```python
from build123d import *

# Parameters (mm, degrees)
F1_DEPTH      = 5
F3_DEPTH      = 10
F5_DEPTH      = 25
F7_R          = 6.7597979746
F6_R          = 2
F8_DEPTH      = 69.4
F9_R          = 5
F10_R         = 5
F11_T1_DEPTH  = 44.2
F11_T3_DEPTH  = 44.2
F12_T1_DEPTH  = 54.4
F12_T3_DEPTH  = 30
F12_T5_DEPTH  = 38
F12_S9_W      = 5
F12_S9_H      = 5
F12_T10_DEPTH = 5
F12_S15_W     = 5
F12_S15_H     = 5
F12_T16_DEPTH = 5
F12_S21_W     = 5
F12_S21_H     = 5
F12_T22_DEPTH = 5
F12_S27_W     = 5
F12_S27_H     = 5
F12_T28_DEPTH = 5
F12_T32_ANGLE = 90
F12_T34_ANGLE = 90


# Not quite as in the source:
# - a fillet or chamfer that OpenCascade refuses, or shapes differently, is made with other operations: its cross-section is extruded or revolved along the edge and cut away or added


with BuildPart() as f1:
    # F0 (on Front) → F1 (new body)
    with BuildSketch(Plane.XZ):
        with BuildLine():
            Line((32.2, -24), (32.2, 24))
            Line((32.2, 24), (8, 24))
            Line((8, 24), (8, 10.8))
            Line((8, 10.8), (8.4, 10.8))
            Line((8.4, 10.8), (8.4, 14.8))
            ThreePointArc((8.4, 14.8), (14.9, 21.3), (21.4, 14.8))
            Line((21.4, 14.8), (21.4, 10.8))
            Line((21.4, 10.8), (24.4, 10.8))
            Line((24.4, 10.8), (24.4, -10.8))
            Line((24.4, -10.8), (21.4, -10.8))
            Line((21.4, -10.8), (21.4, -14.8))
            ThreePointArc((21.4, -14.8), (14.9, -21.3), (8.4, -14.8))
            Line((8.4, -14.8), (8.4, -10.8))
            Line((8.4, -10.8), (-8.4, -10.8))
            Line((-8.4, -10.8), (-8.4, -14.8))
            ThreePointArc((-8.4, -14.8), (-14.9, -21.3), (-21.4, -14.8))
            Line((-21.4, -14.8), (-21.4, -10.8))
            Line((-21.4, -10.8), (-24.4, -10.8))
            Line((-24.4, -10.8), (-24.4, 10.8))
            Line((-24.4, 10.8), (-21.4, 10.8))
            Line((-21.4, 10.8), (-21.4, 14.8))
            ThreePointArc((-21.4, 14.8), (-14.9, 21.3), (-8.4, 14.8))
            Line((-8.4, 14.8), (-8.4, 10.8))
            Line((-8.4, 10.8), (-8, 10.8))
            Line((-8, 10.8), (-8, 24))
            Line((-8, 24), (-32.2, 24))
            Line((-32.2, 24), (-32.2, -24))
            Line((-32.2, -24), (32.2, -24))
        make_face()
    extrude(amount=F1_DEPTH)

    # F2 (on face) → F3 (join)
    with BuildSketch(Plane(origin=(0, 0, 0), x_dir=(-1, 0, 0), z_dir=(0, 1, 0))):
        with BuildLine():
            Line((24.4, 10.8), (24.4, -10.8))
            Line((24.4, -10.8), (21.4, -10.8))
            Line((21.4, -10.8), (21.4, -14.8))
            ThreePointArc((21.4, -14.8), (14.9, -21.3), (8.4, -14.8))
            Line((8.4, -14.8), (8.4, -10.8))
            Line((8.4, -10.8), (-8.4, -10.8))
            Line((-8.4, -10.8), (-8.4, -14.8))
            ThreePointArc((-8.4, -14.8), (-14.9, -21.3), (-21.4, -14.8))
            Line((-21.4, -14.8), (-21.4, -10.8))
            Line((-21.4, -10.8), (-24.4, -10.8))
            Line((-24.4, -10.8), (-24.4, 10.8))
            Line((-24.4, 10.8), (-21.4, 10.8))
            Line((-21.4, 10.8), (-21.4, 14.8))
            ThreePointArc((-21.4, 14.8), (-14.9, 21.3), (-8.4, 14.8))
            Line((-8.4, 14.8), (-8.4, 10.8))
            Line((-8.4, 10.8), (-8, 10.8))
            Line((-8, 10.8), (-8, 24))
            Line((-8, 24), (-32.2, 24))
            Line((-32.2, 24), (-32.2, -24))
            Line((-32.2, -24), (32.2, -24))
            Line((32.2, -24), (32.2, 24))
            Line((32.2, 24), (8, 24))
            Line((8, 24), (8, 10.8))
            Line((8, 10.8), (8.4, 10.8))
            Line((8.4, 10.8), (8.4, 14.8))
            ThreePointArc((8.4, 14.8), (14.9, 21.3), (21.4, 14.8))
            Line((21.4, 14.8), (21.4, 10.8))
            Line((21.4, 10.8), (24.4, 10.8))
        make_face()
        with BuildLine():
            Line((21.4, -14.8), (21.4, -10.8))
            Line((21.4, -10.8), (8.4, -10.8))
            Line((8.4, -10.8), (8.4, -14.8))
            ThreePointArc((8.4, -14.8), (14.9, -21.3), (21.4, -14.8))
        make_face()
        with BuildLine():
            Line((-8.4, -14.8), (-8.4, -10.8))
            Line((-8.4, -10.8), (-21.4, -10.8))
            Line((-21.4, -10.8), (-21.4, -14.8))
            ThreePointArc((-21.4, -14.8), (-14.9, -21.3), (-8.4, -14.8))
        make_face()
        with BuildLine():
            Line((8.4, 10.8), (21.4, 10.8))
            Line((21.4, 10.8), (21.4, 14.8))
            ThreePointArc((21.4, 14.8), (14.9, 21.3), (8.4, 14.8))
            Line((8.4, 14.8), (8.4, 10.8))
        make_face()
        with BuildLine():
            Line((-21.4, 10.8), (-8.4, 10.8))
            Line((-8.4, 10.8), (-8.4, 14.8))
            ThreePointArc((-8.4, 14.8), (-14.9, 21.3), (-21.4, 14.8))
            Line((-21.4, 14.8), (-21.4, 10.8))
        make_face()
    extrude(amount=F3_DEPTH)

    # F4 (on face) → F5 (join)
    with BuildSketch(Plane(origin=(0, 10, 0), x_dir=(-1, 0, 0), z_dir=(0, 1, 0))):
        Polygon((32.2, -24), (32.2, 24), (8, 24), (8, 10.8), (24.4, 10.8), (24.4, -10.8), (-24.4, -10.8), (-24.4, 10.8), (-8, 10.8), (-8, 24), (-32.2, 24), (-32.2, -24), align=None)
        Polygon((8, 10.8), (8, 24), (-8, 24), (-8, 10.8), (-24.4, 10.8), (-24.4, -10.8), (24.4, -10.8), (24.4, 10.8), align=None)
        with BuildLine():
            ThreePointArc((5.5288725662, 5.5), (16.8680666762, 9.6842239514), (24.1, 0))
            ThreePointArc((24.1, 0), (16.8680666762, -9.6842239514), (5.5288725662, -5.5))
            Line((5.5288725662, -5.5), (0, -5.5))
            Line((0, -5.5), (-5.5288725662, -5.5))
            ThreePointArc((-5.5288725662, -5.5), (-24.1, 0), (-5.5288725662, 5.5))
            Line((-5.5288725662, 5.5), (0, 5.5))
            Line((0, 5.5), (5.5288725662, 5.5))
        make_face(mode=Mode.SUBTRACT)
    extrude(amount=F5_DEPTH)

    # F7
    f7_edges = [f1.edges().sort_by_distance(p)[0] for p in [
        (0, 35, 24),
    ]]
    fillet(f7_edges, radius=F7_R)

    # F6 (on face) → F8 (cut)
    with BuildSketch(Plane(origin=(-32.2, 0, 0), x_dir=(0, -1, 0), z_dir=(-1, 0, 0))):
        with Locations((-14, 17.0717967697)):
            Circle(F6_R)
    extrude(amount=-F8_DEPTH, mode=Mode.SUBTRACT)

    # F9
    f9_edges = [f1.edges().sort_by_distance(p)[0] for p in [
        (32.2, 33.020101, 22.020101),
        (32.2, 35, -3.379899),
    ]]
    fillet(f9_edges, radius=F9_R)

    # F10
    f10_edges = [f1.edges().sort_by_distance(p)[0] for p in [
        (-32.2, 35, -3.379899),
    ]]
    fillet(f10_edges, radius=F10_R)

    # F11: fillet of radius 5 on 2 edges, made by hand

    # F11_s2 → F11_t1 (cut)
    with BuildSketch(Plane.YZ.offset(-39.7)):
        with BuildLine():
            ThreePointArc((-5, 19), (-3.5355339059, 22.5355339059), (0, 24))
            Line((0, 24), (-5, 24))
            Line((-5, 24), (-5, 19))
        make_face()
    extrude(amount=F11_T1_DEPTH, mode=Mode.SUBTRACT)

    # F11_s4 → F11_t3 (cut)
    with BuildSketch(Plane.YZ.offset(-4.5)):
        with BuildLine():
            ThreePointArc((-5, 19), (-3.5355339059, 22.5355339059), (0, 24))
            Line((0, 24), (-5, 24))
            Line((-5, 24), (-5, 19))
        make_face()
    extrude(amount=F11_T3_DEPTH, mode=Mode.SUBTRACT)

    # F12: fillet of radius 5 on 8 edges, made by hand

    # F12_s2 → F12_t1 (cut)
    with BuildSketch(Plane.YZ.offset(-27.2)):
        with BuildLine():
            ThreePointArc((30, -24), (33.5355339059, -22.5355339059), (35, -19))
            Line((35, -19), (35, -24))
            Line((35, -24), (30, -24))
        make_face()
        with BuildLine():
            ThreePointArc((-5, -19), (-3.5355339059, -22.5355339059), (0, -24))
            Line((0, -24), (-5, -24))
            Line((-5, -24), (-5, -19))
        make_face()
    extrude(amount=F12_T1_DEPTH, mode=Mode.SUBTRACT)

    # F12_s4 → F12_t3 (cut)
    with BuildSketch(Plane.XZ.offset(-30)):
        with BuildLine():
            ThreePointArc((-27.2, -24), (-30.7355339059, -22.5355339059), (-32.2, -19))
            Line((-32.2, -19), (-32.2, -24))
            Line((-32.2, -24), (-27.2, -24))
        make_face()
        with BuildLine():
            ThreePointArc((32.2, -19), (30.7355339059, -22.5355339059), (27.2, -24))
            Line((27.2, -24), (32.2, -24))
            Line((32.2, -24), (32.2, -19))
        make_face()
    extrude(amount=F12_T3_DEPTH, mode=Mode.SUBTRACT)

    # F12_s6 → F12_t5 (cut)
    with BuildSketch(Plane.XY.offset(-19)):
        with BuildLine():
            ThreePointArc((27.2, -5), (30.7355339059, -3.5355339059), (32.2, 0))
            Line((32.2, 0), (32.2, -5))
            Line((32.2, -5), (27.2, -5))
        make_face()
        with BuildLine():
            ThreePointArc((-27.2, -5), (-30.7355339059, -3.5355339059), (-32.2, 0))
            Line((-32.2, 0), (-32.2, -5))
            Line((-32.2, -5), (-27.2, -5))
        make_face()
    extrude(amount=F12_T5_DEPTH, mode=Mode.SUBTRACT)


with BuildPart() as f12_tool8:
    # F12_s9 → F12_t10 (new body)
    with BuildSketch(Plane.XZ):
        with Locations((-29.7, 21.5)):
            Rectangle(F12_S9_W, F12_S9_H)
    extrude(amount=F12_T10_DEPTH)

    # F12_s11 → F12_t12 (revolve, cut)
    with BuildSketch(Plane(origin=(-27.2, 0, 19), x_dir=(0.7071067812, 0, -0.7071067812), z_dir=(-0.7071067812, 0, -0.7071067812))):
        with BuildLine():
            ThreePointArc((0, -5), (5, 0), (0, 5))
            Line((0, 5), (0, -5))
        make_face()
    revolve(axis=Axis((-27.2, 0, 19), (0, -1, 0)), mode=Mode.SUBTRACT)


with BuildPart() as f1_1:
    add(f1.part)

    # F12_t7: cut F12_tool8
    add(f12_tool8.part, mode=Mode.SUBTRACT)


with BuildPart() as f12_tool14:
    # F12_s15 → F12_t16 (new body)
    with BuildSketch(Plane.XZ):
        with Locations((29.7, 21.5)):
            Rectangle(F12_S15_W, F12_S15_H)
    extrude(amount=F12_T16_DEPTH)

    # F12_s17 → F12_t18 (revolve, cut)
    with BuildSketch(Plane(origin=(27.2, 0, 19), x_dir=(-0.7071067812, 0, -0.7071067812), z_dir=(-0.7071067812, 0, 0.7071067812))):
        with BuildLine():
            ThreePointArc((0, -5), (5, 0), (0, 5))
            Line((0, 5), (0, -5))
        make_face()
    revolve(axis=Axis((27.2, 0, 19), (0, -1, 0)), mode=Mode.SUBTRACT)


with BuildPart() as f1_2:
    add(f1_1.part)

    # F12_t13: cut F12_tool14
    add(f12_tool14.part, mode=Mode.SUBTRACT)


with BuildPart() as f12_tool20:
    # F12_s21 → F12_t22 (new body)
    with BuildSketch(Plane.XZ):
        with Locations((-29.7, -21.5)):
            Rectangle(F12_S21_W, F12_S21_H)
    extrude(amount=F12_T22_DEPTH)

    # F12_s23 → F12_t24 (revolve, cut)
    with BuildSketch(Plane(origin=(-27.2, 0, -19), x_dir=(0.7071067812, 0, 0.7071067812), z_dir=(0.7071067812, 0, -0.7071067812))):
        with BuildLine():
            ThreePointArc((0, -5), (5, 0), (0, 5))
            Line((0, 5), (0, -5))
        make_face()
    revolve(axis=Axis((-27.2, 0, -19), (0, -1, 0)), mode=Mode.SUBTRACT)


with BuildPart() as f1_3:
    add(f1_2.part)

    # F12_t19: cut F12_tool20
    add(f12_tool20.part, mode=Mode.SUBTRACT)


with BuildPart() as f12_tool26:
    # F12_s27 → F12_t28 (new body)
    with BuildSketch(Plane.XZ):
        with Locations((29.7, -21.5)):
            Rectangle(F12_S27_W, F12_S27_H)
    extrude(amount=F12_T28_DEPTH)

    # F12_s29 → F12_t30 (revolve, cut)
    with BuildSketch(Plane(origin=(27.2, 0, -19), x_dir=(-0.7071067812, 0, 0.7071067812), z_dir=(0.7071067812, 0, 0.7071067812))):
        with BuildLine():
            ThreePointArc((0, -5), (5, 0), (0, 5))
            Line((0, 5), (0, -5))
        make_face()
    revolve(axis=Axis((27.2, 0, -19), (0, -1, 0)), mode=Mode.SUBTRACT)


with BuildPart() as f1_4:
    add(f1_3.part)

    # F12_t25: cut F12_tool26
    add(f12_tool26.part, mode=Mode.SUBTRACT)

    # F12_s31 → F12_t32 (revolve, cut)
    with BuildSketch(Plane.XZ.offset(-30)):
        with BuildLine():
            ThreePointArc((-27.2, -24), (-30.7355339059, -22.5355339059), (-32.2, -19))
            Line((-32.2, -19), (-32.2, -24))
            Line((-32.2, -24), (-27.2, -24))
        make_face()
    revolve(axis=Axis((-27.2, 30, -24), (0, 0, -1)), revolution_arc=F12_T32_ANGLE, mode=Mode.SUBTRACT)

    # F12_s33 → F12_t34 (revolve, cut)
    with BuildSketch(Plane.XZ.offset(-30)):
        with BuildLine():
            ThreePointArc((27.2, -24), (30.7355339059, -22.5355339059), (32.2, -19))
            Line((32.2, -19), (32.2, -24))
            Line((32.2, -24), (27.2, -24))
        make_face()
    revolve(axis=Axis((27.2, 30, -24), (0, 0, 1)), revolution_arc=F12_T34_ANGLE, mode=Mode.SUBTRACT)


solid = f1_4.part
```
Verification items for the finished model (mm, model axes). A direction names the side the tool comes from. Round coordinates to 2 decimals unless told otherwise and drop trailing zeros. Order: outer loops, then holes, each group sorted by start corner. A loop starts at its lowest first (then second) coordinate and runs counter-clockwise, first axis right, second up. Notation, with made-up numbers: (63, 40) -> (68, 40) arc R16 ccw to (68, 57) -> close; hole circle Ø11 at (8.5, 87.5). An arc over 180 degrees is marked (long way). Put each result on its own line as item: value. Start each with the question number.
(1) Tool access check on faces 1 (the face through (-30.7, -3.57, -0.27)), 2 (the face through (15, -2.5, -21.3)), 3 (the face through (-8, 2, 17)), 4 (the face through (0, 22, -5.5)), 5 (the face through (-8.3, -5, 16.1)). Record the directions out of +Z, -Z, +X, -X, +Y, -Y that give a thin tool (end or side, any length) a straight path to the whole face; none if there is none.
(2) Draft check along Z on faces 6 (the face through (0, 33, -23)), 7 (the face through (24.093, 22.325, -0.363)), 8 (the face through (32.2, 15, 0)), 9 (the face through (-18, -4, 22)). Enter one of: +Z half, -Z half, draft (parallel to the pull), parting line (faces both ways), or undercut.
(3) Section check B-B (y = 17.5). Enter the section's corners in (x, z), then the cut area to 3 significant figures.
(4) Section check C-C (z = -2.5). Enter the section's corners in (x, y).
(5) Section check A-A (x = 14). Enter the section's corners in (y, z).
(6) Depth check by flat-ended pin: pin 1 Ø2 at (y, z) = (-3, -12) entering from -X; pin 2 Ø6 at (x, y) = (4.5, 0.5) entering from +Z; pin 3 Ø5 at (x, z) = (-14, 16.5) entering from -Y. Enter the tip coordinate at first touch or a pass-through.
(7) Section check D-D (y = 7.5). Enter the section's corners in (x, z), then the cut area to 3 significant figures.
(8) Material ranges on line 1 along Z through (x, y) = (5.5, 14); line 2 along Z through (x, y) = (-18, 9); line 3 along X through (y, z) = (26, 0), recorded low to high.
Completed:
1. face 1: +Z, -Z, -X, -Y
1. face 2: -Y
1. face 3: +Z, -Y
1. face 4: +Y, -Y
1. face 5: +Z, -Z, +X, -X, -Y
2. face 6: -Z half
2. face 7: undercut
2. face 8: draft
2. face 9: +Z half
3. outline: (-32.2, -19) arc R5 ccw to (-27.2, -24) -> (27.2, -24) arc R5 ccw to (32.2, -19) -> (32.2, 19) arc R5 ccw to (27.2, 24) -> (-27.2, 24) arc R5 ccw to (-32.2, 19) -> close; hole (-5.53, -5.5) -> (5.53, -5.5) arc R10.1 ccw (long way) to (5.53, 5.5) -> (-5.53, 5.5) arc R10.1 ccw (long way) to start
3. area: 2,330 mm2
4. outline: (-32.2, 0) arc R5 ccw to (-27.2, -5) -> (-24.4, -5) -> (-24.4, 10) -> (-23.79, 10) -> (-23.79, 35) -> (-27.2, 35) arc R5 ccw to (-32.2, 30) -> close; (23.79, 10) -> (24.4, 10) -> (24.4, -5) -> (27.2, -5) arc R5 ccw to (32.2, 0) -> (32.2, 30) arc R5 ccw to (27.2, 35) -> (23.79, 35) -> close
5. outline: (-4.47, -21.24) arc R5 ccw to (0, -24) -> (30, -24) arc R5 ccw to (35, -19) -> (35, -10.1) -> (10, -10.1) -> (10, -10.8) -> (0, -10.8) -> (0, -21.24) -> close; (-4.47, 21.24) -> (0, 21.24) -> (0, 10.8) -> (10, 10.8) -> (10, 10.1) -> (35, 10.1) -> (35, 17.24) arc R6.76 ccw to (28.24, 24) -> (0, 24) arc R5 ccw to start; hole circle Ø4 at (14, 17.07)
6. pin 1: stops at x = -31.78
6. pin 2: stops at z = -10.8
6. pin 3: stops at y = 0
7. outline: (-32.2, -19) arc R5 ccw to (-27.2, -24) -> (27.2, -24) arc R5 ccw to (32.2, -19) -> (32.2, 19) arc R5 ccw to (27.2, 24) -> (8, 24) -> (8, 10.8) -> (24.4, 10.8) -> (24.4, -10.8) -> (-24.4, -10.8) -> (-24.4, 10.8) -> (-8, 10.8) -> (-8, 24) -> (-27.2, 24) arc R5 ccw to (-32.2, 19) -> close
7. area: 1,800 mm2
8. line 1: z = -24 to -5.5, 5.5 to 15.07, 19.07 to 24
8. line 2: z = -24 to -10.8, 10.8 to 24
8. line 3: x = -32.2 to -24.1, 24.1 to 32.2
